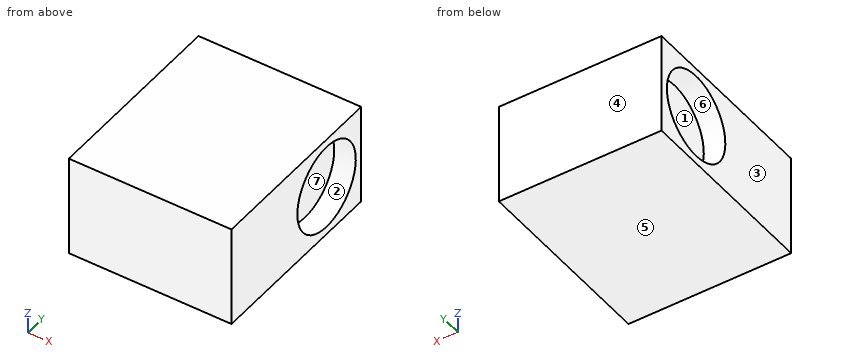
from build123d import *

# Parameters (mm, degrees)
SKETCH1_W           = 37.8
SKETCH1_H           = 44.4
BOSS_EXTRUDE1_DEPTH = 23.7
SKETCH2_R           = 10
CUT_EXTRUDE1_DEPTH  = 5


with BuildPart() as part:
    # Sketch1 → Boss-Extrude1 (new body)
    with BuildSketch(Plane.XY):
        with Locations((15.249090909, -6.911818182)):
            Rectangle(SKETCH1_W, SKETCH1_H)
    extrude(amount=BOSS_EXTRUDE1_DEPTH)

    # Sketch2 → Cut-Extrude1 (cut)
    with BuildSketch(Plane(origin=(34.149090909, 0, 0), x_dir=(0, 0, -1), z_dir=(1, 0, 0))):
        with Locations((-11.85, 3.438181818)):
            Circle(SKETCH2_R)
    cut_extrude1 = extrude(amount=-CUT_EXTRUDE1_DEPTH, mode=Mode.SUBTRACT)

    # Mirror1: Cut-Extrude1 across plane
    add(cut_extrude1.mirror(Plane(origin=(15.249090909, 0, 0), x_dir=(0, 0, 1), z_dir=(1, 0, 0))), mode=Mode.SUBTRACT)


solid = part.part
Work out the finished part from the listing and answer in its coordinate system (mm). Face numbers are marked on the shaded views. A direction names the side the tool comes from. Give positions to 0.01 mm unless a question says otherwise; leave off trailing zeros. Loops run counter-clockwise (first coordinate to the right, second up) from the corner with the lowest first, then second, coordinate; pieces in that order, holes last. Notation, with made-up numbers: (-23.75, 29.25) - (-17.75, 29.25) arc R24 cw to (-17.75, 61.25) - close; hole circle Ø3 at (-33, -32.5). An arc over 180 degrees is marked (long way). Answer in a Markdown table with one row per item.
(1) Section B-B (y = -0.5) is taken. Give the vertices of the cut face in (x, z), and give its area (3 significant figures).
Results list:
| item | result |
|---|---|
| outline | (-3.65, 0) - (34.15, 0) - (34.15, 2.66) - (29.15, 2.66) - (29.15, 21.04) - (34.15, 21.04) - (34.15, 23.7) - (-3.65, 23.7) - (-3.65, 21.04) - (1.35, 21.04) - (1.35, 2.66) - (-3.65, 2.66) - close |
| area | 712 mm² |
(2) For a pull along Z with two mould halves and no side action, classify the marked faces 4, 5, 6 and 7 as pulls with the +Z half, pulls with the -Z half, needs draft (parallel to the pull), parting line crosses it, or undercut.
Results list:
| item | result |
|---|---|
| face 4 | needs draft |
| face 5 | pulls with the -Z half |
| face 6 | undercut |
| face 7 | undercut |
(3) Section C-C (x = -0.5) is taken. Give the vertices of the cut face in (y, z), and give its area (3 significant figures).
Results list:
| item | result |
|---|---|
| outline | (-29.11, 0) - (15.29, 0) - (15.29, 23.7) - (-29.11, 23.7) - close; hole circle Ø20 at (3.44, 11.85) |
| area | 738 mm² |
(4) Flat-ended cylindrical pins translate along their axes: pin 1 Ø2 at (y, z) = (-3, 6.5) entering from +X; pin 2 Ø12 at (y, z) = (3.44, 11.85) entering from -X. Find the tip coordinate at first contact, or state that the pin passes through.
Results list:
| item | result |
|---|---|
| pin 1 | stops at x = 29.15 |
| pin 2 | stops at x = 1.35 |
(5) Consider L1, parallel to Y at x = 30.9, z = 11.85; L2, parallel to X at y = 0.5, z = 6.25; L3, parallel to Y at x = 32, z = 8. Determine where each line is inside the solid, lowest interval first. Write a range as [from, to].
Results list:
| item | result |
|---|---|
| L1 | y = [-29.11, -6.56], [13.44, 15.29] |
| L2 | x = [1.35, 29.15] |
| L3 | y = [-29.11, -5.79], [12.67, 15.29] |
(6) A tool of negligible diameter and unlimited length cuts with its end or side. For the marked faces 1, 2 and 3, from which of +Z, -Z, +X, -X, +Y, -Y can it reach the whole face along a straight path? Write none if from no direction.
Results list:
| item | result |
|---|---|
| face 1 | -X |
| face 2 | +X |
| face 3 | +Z, -Z, -X, +Y, -Y |
(7) Section A-A (z = 11.85) is taken. Give the vertices of the cut face in (x, y), and give its area (3 significant figures).
Results list:
| item | result |
|---|---|
| outline | (-3.65, -29.11) - (34.15, -29.11) - (34.15, -6.56) - (29.15, -6.56) - (29.15, 13.44) - (34.15, 13.44) - (34.15, 15.29) - (-3.65, 15.29) - (-3.65, 13.44) - (1.35, 13.44) - (1.35, -6.56) - (-3.65, -6.56) - close |
| area | 1,480 mm² |
